Geometry: final body of the model. Coordinates: model frame, mm. A direction names the side the tool comes from. Coordinates: 2 decimals unless noted, no trailing zeros. Order: outer loops, then holes, each group sorted by start corner. A loop starts at its lowest first (then second) coordinate and runs counter-clockwise, first axis right, second up. Notation, with made-up numbers: M -26.75,-36 L -8.75,-36 A18 cw -8.75,-14 Z; hole C 33.5,24 d2. An arc over 180 degrees is marked long. Use CSV: the item, a comma, the result in double quotes. Start each with the question number.
1. Section query A-A on z = 30.5. Return the cut outline in (x, y).
2. Section query D-D on z = 53. Return the cut outline in (x, y).
3. Section query C-C on x = 94. Return the cut outline in (y, z), and give its area (3 significant figures).
4. Set-up query: faces 5 (the flat face through (-53, -17.597, 64)), 6 (the flat face through (-54, 45, 76.2)), 7 (the flat face through (42, -52.54, 18)). Return all of +Z, -Z, +X, -X, +Y, -Y with unobstructed straight access to the full face (end or side cutting, diameter ignored); none if empty.
5. First-contact query: P1, Ø12, axis at x = 46.5, y = -11.41, coming from the +Z side; P2, Ø3, axis at x = 33.5, z = 44, coming from the -Y side; P3, Ø18, axis at x = 46.5, y = 45.14, coming from the -Z side; P4, Ø4, axis at y = -62, z = 47.5, coming from the +X side. Flat tips, straight axial feed; report the tip coordinate or a pass-through.
6. Material intervals for line 1 (Y direction, x = -43.5, z = 64); line 2 (Y direction, x = 42, z = 43.5); line 3 (Y direction, x = 50.5, z = 15), sorted ascending.
7. Section query B-B on y = 42. Return the cut outline in (x, z).
8. Pull-direction query (X, two-part tool) for faces 1 (the cylindrical face through (85.943, 45.478, 5.889)), 2 (the flat face through (-107.337, -1, 38)), 3 (the flat face through (-46, -65.24, 38)), 4 (the flat face through (52.92, -0.91, 38.63)); classes: pulls with the +X half, pulls with the -X half, needs draft (parallel to the pull), parting line crosses it, or undercut.
from build123d import *

# Parameters (mm, degrees)
F0_W      = 214.6737128496
F0_H      = 130.4792463779
F1_DEPTH  = 76.2
F3_DEPTH  = 2540
F4_W      = 107.3368564248
F4_H      = 42.1587638557
F5_DEPTH  = 25.4
F6_W      = 42.1587638557
F6_H      = 25.4
F7_DEPTH  = 25.4
F8_DEPTH  = 25.4
F10_DEPTH = 12.7
F11_R     = 7.7814226796
F11_R_2   = 7.6137292191
F12_DEPTH = 76.201


with BuildPart() as f1:
    # F0 (on Top) → F1 (new body)
    with BuildSketch(Plane.XY):
        Rectangle(F0_W, F0_H)
    extrude(amount=F1_DEPTH)

    # F2 (on face) → F3 (cut)
    with BuildSketch(Plane.XZ.offset(65.239623189)):
        Polygon((107.3368564248, 76.2), (0, 76.2), (107.3368564248, 0), align=None)
    extrude(amount=-F3_DEPTH, mode=Mode.SUBTRACT)

    # F4 (on face) → F5 (cut)
    with BuildSketch(Plane.XY.offset(76.2)):
        with Locations((-53.6684282124, 3.4826807678)):
            Rectangle(F4_W, F4_H)
    extrude(amount=-F5_DEPTH, mode=Mode.SUBTRACT)

    # F6 (on face) → F7 (cut)
    with BuildSketch(Plane(origin=(0, 0, 0), x_dir=(0, -1, 0), z_dir=(-1, 0, 0))):
        with Locations((-3.4826807678, 63.5)):
            Rectangle(F6_W, F6_H)
    extrude(amount=-F7_DEPTH, mode=Mode.SUBTRACT)

    # F8 (cut): a face of the model
    f8_faces = [f1.faces().sort_by_distance(p)[0] for p in [
        (25.4, 3.4826807678, 54.4840847568),
    ]]
    extrude(f8_faces, amount=-F8_DEPTH, mode=Mode.SUBTRACT)

    # F9 (on face) → F10 (cut)
    with BuildSketch(Plane.XZ.offset(65.239623189)):
        Polygon((107.3368564248, 0), (17.6323605159, 63.6825300827), (17.6323605159, 0), align=None)
    extrude(amount=-F10_DEPTH, mode=Mode.SUBTRACT)

    # F11 (on Top) → F12 (cut, through all)
    with BuildSketch(Plane.XY):
        with Locations((46.5043671429, 45.1353924804)):
            Circle(F11_R)
        with Locations((46.5043671429, -11.4098191261)):
            Circle(F11_R_2)
        with Locations((93.7171405072, -11.4098191261)):
            Circle(F11_R_2)
        with Locations((93.7171405072, 45.1353924804)):
            Circle(F11_R)
    extrude(amount=F12_DEPTH, mode=Mode.SUBTRACT)


solid = f1.part
Results list:
1,outline,"M -107.34,-65.24 L 17.63,-65.24 L 17.63,-52.54 L 64.37,-52.54 L 64.37,65.24 L -107.34,65.24 Z; hole C 46.5,45.14 d15.56; hole C 46.5,-11.41 d15.23"
2,outline,"M -107.34,-65.24 L 17.63,-65.24 L 17.63,-52.54 L 32.68,-52.54 L 32.68,-17.6 L -107.34,-17.6 Z; M -107.34,24.56 L 32.68,24.56 L 32.68,65.24 L -107.34,65.24 Z"
3,outline,"M -52.54,0 L -19.02,0 L -19.02,9.47 L -52.54,9.47 Z; M -3.8,0 L 37.36,0 L 37.36,9.47 L -3.8,9.47 Z; M 52.91,0 L 65.24,0 L 65.24,9.47 L 52.91,9.47 Z"
3,area,"824 mm²"
4,face 5,"+Z, +X, -X"
4,face 6,"+Z, +X, -X, +Y, -Y"
4,face 7,"+Z, -Z, +X, -Y"
5,P1,"passes through"
5,P2,"stops at y = -52.54"
5,P3,"stops at z = 0"
5,P4,"stops at x = 17.63"
6,line 1,"y = -65.24 to -17.6, 24.56 to 65.24"
6,line 2,"y = -52.54 to -17.55, -5.27 to 38.79, 51.48 to 65.24"
6,line 3,"y = -52.54 to -17.89, -4.93 to 38.46, 51.81 to 65.24"
7,outline,"M -107.34,0 L 39.38,0 L 39.38,48.24 L 0,76.2 L -107.34,76.2 Z; M 53.63,0 L 86.6,0 L 86.6,14.72 L 53.63,38.13 Z; M 100.84,0 L 107.34,0 L 100.84,4.61 Z"
8,face 1,"undercut"
8,face 2,"pulls with the -X half"
8,face 3,"needs draft"
8,face 4,"pulls with the +X half"
